Build history of the part. All positions in model axes, mm. A direction names the side the tool comes from. Coordinates: 2 decimals unless noted, no trailing zeros. Write each loop counter-clockwise with the first axis right and the second up, starting at its lowest first coordinate (ties: lowest second). Pieces come first, ordered by that corner, then holes. Notation, with made-up numbers: M 55.5,38.25 L 87.5,38.25 A25 cw 87.5,64.25 Z; hole C -19,18.5 d8. An arc over 180 degrees is marked long. Use CSV: the item, a comma, the result in double quotes. Start each with the question number.
```python
from build123d import *

# Parameters (mm, degrees)
F1_DEPTH = 100


with BuildPart() as f1:
    # F0 (on Front) → F1 (new body)
    with BuildSketch(Plane.XZ):
        Polygon((-70, -17.953758), (-110, -17.953758), (-110, -32.953758), (40, -32.953758), (40, -17.953758), (0, -17.953758), align=None)
        with BuildLine():
            Line((-70, 82.046242), (-70, -17.953758))
            Line((-70, -17.953758), (0, -17.953758))
            Line((0, -17.953758), (0, 82.046242))
            Line((0, 82.046242), (-5, 82.046242))
            ThreePointArc((-5, 82.046242), (-35, 52.046242), (-65, 82.046242))
            Line((-65, 82.046242), (-70, 82.046242))
        make_face()
    extrude(amount=F1_DEPTH)


solid = f1.part
```
1. Flat gauge pins, fed straight in: pin 1 (20 mm diameter, centred on x = 26.5, y = -28, fed in from +Z); pin 2 (5 mm diameter, centred on y = -57, z = 2, fed in from +X); pin 3 (10 mm diameter, centred on x = -57.5, y = -58.5, fed in from +Z). Where does each tip first touch, or does it go through?
2. Slice it at B-B (z = 28.5). List the corners of the cut face in (x, y).
3. 3-axis set-ups, long thin cutter, end or side, ignore diameter. For faces 1 (the flat face through (-70, -49, 33)), 2 (the flat face through (-36, -100, 13)), 3 (the flat face through (20, -49, -17.954)): which of +Z, -Z, +X, -X, +Y, -Y reach the whole face in a straight line?
4. Slice it at A-A (y = -13). List the corners of the cut face in (x, z), and give its area (3 significant figures).
5. Drill centre lines: line 1 along X through (y, z) = (-19, -12); line 2 along Z through (x, y) = (-98, -35.5); line 3 along X through (y, z) = (-5, 70.5). Where is each one in solid material? Low to high. Write a range as from..to.
6. Slice it at C-C (x = -35). List the corners of the cut face in (y, z).
Established:
1,pin 1,"stops at z = -17.95"
1,pin 2,"stops at x = 0"
1,pin 3,"stops at z = 70.06"
2,outline,"M -70,-100 L 0,-100 L 0,0 L -70,0 Z"
3,face 1,"+Z, -X, +Y, -Y"
3,face 2,"+Z, -Z, +X, -X, -Y"
3,face 3,"+Z, +X, +Y, -Y"
4,outline,"M -110,-32.95 L 40,-32.95 L 40,-17.95 L 0,-17.95 L 0,82.05 L -5,82.05 A30 cw -65,82.05 L -70,82.05 L -70,-17.95 L -110,-17.95 Z"
4,area,"7,840 mm2"
5,line 1,"x = -70..0"
5,line 2,"z = -32.95..-17.95"
5,line 3,"x = -70..-62.69, -7.31..0"
6,outline,"M -100,-32.95 L 0,-32.95 L 0,52.05 L -100,52.05 Z"
